The listing builds one solid part. Answer for the finished solid, in the listing's coordinates (mm). Face numbers are marked on the shaded views. A direction names the side the tool comes from. Coordinates: 2 decimals unless noted, no trailing zeros. Write each loop counter-clockwise with the first axis right and the second up, starting at its lowest first coordinate (ties: lowest second). Pieces come first, ordered by that corner, then holes.
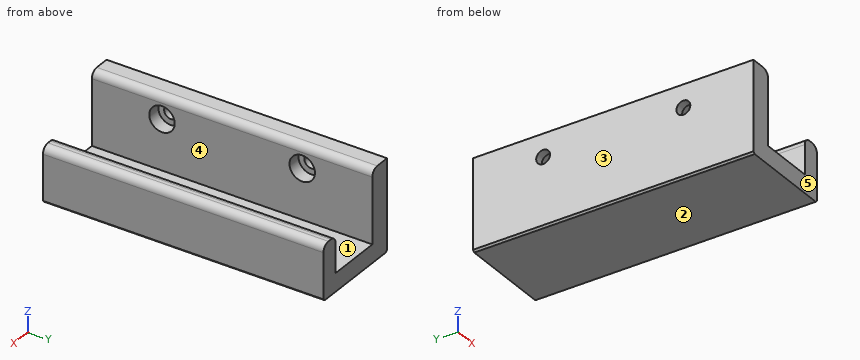
from build123d import *

# Parameters (mm, degrees)
F0_W           = 7.5
F0_H           = 5
F1_DEPTH       = 38.5
F3_D           = 3.8
F3_DEPTH       = 6
F3_CBORE_D     = 7
F3_CBORE_DEPTH = 3.7
F4_R           = 2
F5_SIZE        = 0.5


with BuildPart() as f1:
    # F0 (on Front) → F1 (new body, symmetric)
    with BuildSketch(Plane.XZ):
        with Locations((3.75, 2.5)):
            Rectangle(F0_W, F0_H)
        with Locations((-3.75, 2.5)):
            Rectangle(F0_W, F0_H)
        Polygon((7.5, 5), (7.5, 0), (12.5, 0), (12.5, 15), (7.5, 15), align=None)
        Polygon((-13.5, 0), (-7.5, 0), (-7.5, 5), (-7.5, 25), (-13.5, 25), align=None)
    extrude(amount=F1_DEPTH, both=True)

    # F3
    with Locations(Plane.YZ.offset(-7.5)):
        with Locations((-19.25, 18.75), (19.25, 18.75)):
            CounterBoreHole(F3_D / 2, F3_CBORE_D / 2, F3_CBORE_DEPTH, depth=F3_DEPTH)

    # F4
    f4_edges = [f1.edges().sort_by_distance(p)[0] for p in [
        (12.5, 0, 15),
        (7.5, 0, 15),
        (-7.5, 0, 25),
    ]]
    fillet(f4_edges, radius=F4_R)

    # F5
    f5_edges = [f1.edges().sort_by_distance(p)[0] for p in [
        (12.5, 0, 0),
        (-13.5, 0, 0),
    ]]
    chamfer(f5_edges, length=F5_SIZE)


solid = f1.part
1. Section A-A on z = 8.25 is taken. Give the vertices of the cut face in (x, y).
Results found:
outline: (-13.5, -38.5) - (-7.5, -38.5) - (-7.5, 38.5) - (-13.5, 38.5) - close; (7.5, -38.5) - (12.5, -38.5) - (12.5, 38.5) - (7.5, 38.5) - close
2. Section C-C on z = 18.75 is taken. Give the vertices of the cut face in (x, y), then the cut area to 3 significant figures.
Results found:
outline: (-13.5, -38.5) - (-7.5, -38.5) - (-7.5, -22.75) - (-11.2, -22.75) - (-11.2, -21.15) - (-13.5, -21.15) - close; (-13.5, -17.35) - (-11.2, -17.35) - (-11.2, -15.75) - (-7.5, -15.75) - (-7.5, 15.75) - (-11.2, 15.75) - (-11.2, 17.35) - (-13.5, 17.35) - close; (-13.5, 21.15) - (-11.2, 21.15) - (-11.2, 22.75) - (-7.5, 22.75) - (-7.5, 38.5) - (-13.5, 38.5) - close
area: 393 mm2
3. Find the intervals of material crossed by L1, parallel to X at y = -27.5, z = 5.75; L2, parallel to Z at x = -12.7, y = 19.25; L3, parallel to Z at x = -9.8, y = 19.25, in increasing order.
Results found:
L1: x = -13.5 to -7.5, 7.5 to 12.5
L2: z = 0 to 16.85, 20.65 to 25
L3: z = 0 to 15.25, 22.25 to 25
4. Flat-ended cylindrical pins translate along their axes: P1, Ø3.5, axis at y = -19.25, z = 18.75, coming from the +X side; P2, Ø5.5, axis at y = 19.5, z = 19.5, coming from the +X side; P3, Ø3, axis at x = -2.5, y = 8, coming from the +Z side; P4, Ø4.5, axis at y = 19.25, z = 18.75, coming from the +X side. Find the tip coordinate at first contact, or state that the pin passes through.
Results found:
P1: passes through
P2: stops at x = -7.5
P3: stops at z = 5
P4: stops at x = -11.2
5. For a pull along X with two mould halves and no side action, classify the marked faces 1, 2 and 3 as pulls with the +X half, pulls with the -X half, needs draft (parallel to the pull), parting line crosses it, or undercut.
Results found:
face 1: undercut
face 2: needs draft
face 3: pulls with the -X half
6. Section D-D on y = -23.5 is taken. Give the vertices of the cut face in (x, z).
Results found:
outline: (-13.5, 0.5) - (-13, 0) - (12, 0) - (12.5, 0.5) - (12.5, 13) arc R2 ccw to (10.5, 15) - (9.5, 15) arc R2 ccw to (7.5, 13) - (7.5, 5) - (-7.5, 5) - (-7.5, 23) arc R2 ccw to (-9.5, 25) - (-13.5, 25) - close
7. A tool of negligible diameter and unlimited length cuts with its end or side. For the marked faces 4 and 5, from which of +Z, -Z, +X, -X, +Y, -Y can it reach the whole face along a straight path? Write none if from no direction.
Results found:
face 4: +Z, +Y, -Y
face 5: +Z, -Z, +X, -X, -Y
8. Section B-B on y = 19.25 is taken. Give the vertices of the cut face in (x, z).
Results found:
outline: (-13.5, 0.5) - (-13, 0) - (12, 0) - (12.5, 0.5) - (12.5, 13) arc R2 ccw to (10.5, 15) - (9.5, 15) arc R2 ccw to (7.5, 13) - (7.5, 5) - (-7.5, 5) - (-7.5, 15.25) - (-11.2, 15.25) - (-11.2, 16.85) - (-13.5, 16.85) - close; (-13.5, 20.65) - (-11.2, 20.65) - (-11.2, 22.25) - (-7.5, 22.25) - (-7.5, 23) arc R2 ccw to (-9.5, 25) - (-13.5, 25) - close
